Here's how the part is built. I have some questions about the finished solid (model axes, mm). Round coordinates to 2 decimals unless told otherwise and drop trailing zeros. Loops run counter-clockwise (first coordinate to the right, second up) from the corner with the lowest first, then second, coordinate; pieces in that order, holes last. Notation, with made-up numbers: (13, 11) -> (66, 11) arc R17 cw to (66, 37) -> close; hole circle Ø7 at (-21.75, 1.25). An arc over 180 degrees is marked (long way). Use one line per item in the form item = value. Start each with the question number.
Item 1: If we section it at B-B (y = 186.5): Write out the boundary of the cut face in (x, z).
Item 2: I'm going to push flat-ended pins straight in: pin 1 Ø4 at (x, z) = (-5, 17) entering from +Y (3 decimals); pin 2 Ø4.5 at (y, z) = (161.925, 9.525) entering from +X. Where does each tip first touch, or does it pass through?
Item 3: If I drill on L1, parallel to Z at x = -10.75, y = 177.5; L2, parallel to X at y = 701, z = 4, over which ranges is the centre line in solid material (lowest first)? Write a range as [from, to].
Autodesk Inventor part; units mm, degrees
ref_plane "YZ Plane" through (0, 0, 0) normal (1, 0, 0) x (0, 1, 0)
ref_plane "XZ Plane" through (0, 0, 0) normal (0, 1, 0) x (-1, 0, 0)
ref_plane "XY Plane" through (0, 0, 0) normal (0, 0, 1) x (1, 0, 0)
sketch "Sketch1" plane through (0, 0, 0) normal (0, 1, 0) x (-1, 0, 0)
  line L0 (0, 0) -> (19.05, 0)
  line L1 (19.05, 0) -> (19.05, 19.05)
  line L2 (19.05, 19.05) -> (0, 19.05)
  line L3 (0, 19.05) -> (0, 0)
  line L4 (1.5875, 17.4625) -> (17.4625, 17.4625)
  line L5 (17.4625, 17.4625) -> (17.4625, 1.5875)
  line L6 (17.4625, 1.5875) -> (1.5875, 1.5875)
  line L7 (1.5875, 1.5875) -> (1.5875, 17.4625)
  dimension "d0" = 19.05
  dimension "sqAlumWidth" = 19.05
  dimension "sqAlumWallThickness" = 1.5875
  dimension "d3" = 1.5875
  dimension "d4" = 1.5875
  dimension "d5" = 1.5875
extrude "Extrusion1" add sketch "Sketch1" along normal blind 765.175
sketch "Sketch2" plane through (0, 0, 19.05) normal (1, 0, 0) x (0, 0, -1)
  line L0 (0, 0) -> (19.05, 0)
  line L1 (19.05, 0) -> (19.05, 765.175)
  circle A0 centre (9.525, 12.7) radius 2.4805
  circle A1 centre (9.525, 161.925) radius 2.4805
  dimension "d8" = 4.9609
  dimension "d9" = 149.225
  dimension "screwDistanceFromBottom" = 12.7
  dimension "d11" = 9.525
extrude "Extrusion2" cut sketch "Sketch2" against normal through all
equation "\"d0\" = sqAlumWidth"
equation "\"d3\" = sqAlumWallThickness"
equation "\"d4\" = sqAlumWallThickness"
equation "\"d5\" = sqAlumWallThickness"
equation "\"d6\" = heightAboveTv + largeScrewDistance + topLargeScrewDistanceFromTop + screwDistanceFromBottom"
equation "\"d8\" = largeScrewDiameter"
equation "\"d9\" = largeScrewDistance"
equation "\"d11\" = 0.5 * sqAlumWidth"
equation "\"heightAboveTv\" = 304.8"
properties part number "arm-vertical"
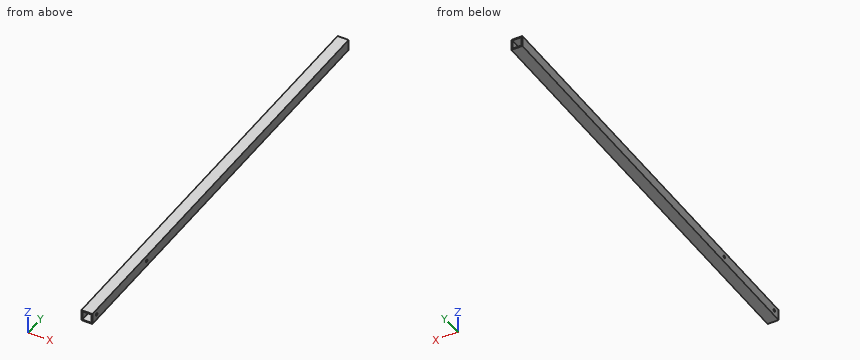
Values found:
q1.outline = (-19.05, 0) -> (0, 0) -> (0, 19.05) -> (-19.05, 19.05) -> close; hole (-17.46, 1.59) -> (-1.59, 1.59) -> (-1.59, 17.46) -> (-17.46, 17.46) -> close
q2.pin_1 = 765.175
q2.pin_2 = through
q3.L1 = [0, 1.59], [17.46, 19.05]
q3.L2 = [-19.05, -17.46], [-1.59, 0]
